from build123d import *

# Parameters (mm, degrees)
BOSS_EXTRU_1_DEPTH     = 200
D_GAGEMENT_M3_52_D     = 4.2
D_GAGEMENT_M3_52_DEPTH = 50
D_GAGEMENT_M3_52_TIP   = 1.2618073


with BuildPart() as part:
    # Esquisse2 → Boss.-Extru.1 (new body)
    with BuildSketch(Plane.XY):
        with BuildLine():
            Line((30, 0), (35, 0))
            Line((35, 0), (35, 10))
            Line((35, 10), (42, 10))
            Line((42, 10), (42, 0))
            Line((42, 0), (50, 0))
            ThreePointArc((50, 0), (35.355339059, 35.355339059), (0, 50))
            Line((0, 50), (0, 42))
            Line((0, 42), (10, 42))
            Line((10, 42), (10, 35))
            Line((10, 35), (0, 35))
            Line((0, 35), (0, 30))
            ThreePointArc((0, 30), (21.213203436, 21.213203436), (30, 0))
        make_face()
    extrude(amount=-BOSS_EXTRU_1_DEPTH)

    # Dégagement M3.52
    with Locations(Plane(origin=(0, 0, -200), x_dir=(-1, 0, 0), z_dir=(0, 0, -1))):
        with Locations((-28.284271247, 28.284271247)):
            Hole(D_GAGEMENT_M3_52_D / 2, depth=D_GAGEMENT_M3_52_DEPTH)
            with Locations((0, 0, -(D_GAGEMENT_M3_52_DEPTH + D_GAGEMENT_M3_52_TIP / 2))):  # 118° drill point
                Cone(0, D_GAGEMENT_M3_52_D / 2, D_GAGEMENT_M3_52_TIP, mode=Mode.SUBTRACT)


solid = part.part
Can you work these out from the model? Positions are in its coordinate system, mm. A direction names the side the tool comes from. Coordinates: 2 decimals unless noted, no trailing zeros. Write each loop counter-clockwise with the first axis right and the second up, starting at its lowest first coordinate (ties: lowest second). Pieces come first, ordered by that corner, then holes.
Q1. If we mould it in two halves opening along Y, with no side actions, what happens to faces 4 (the face through (35.742, 34.964, -98.6)), 5 (the face through (26.736, 29.704, -174.65)), 6 (the face through (38, 10, -99)), 7 (the face through (25, 25, -200))? For each: +Y half, -Y half, draft (parallel to the pull), parting line (faces both ways), or undercut.
Results found:
face 4: +Y half
face 5: undercut
face 6: -Y half
face 7: draft
Q2. Imagine slicing it at C-C, the plane z = -54.5. List the corners of the cut face in (x, y) for me, plus the area to 3 significant figures.
Results found:
outline: (0, 30) arc R30 cw to (30, 0) - (35, 0) - (35, 10) - (42, 10) - (42, 0) - (50, 0) arc R50 ccw to (0, 50) - (0, 42) - (10, 42) - (10, 35) - (0, 35) - close
area: 1,120 mm2
Q3. Imagine slicing it at B-B, the plane z = -153.5. List the corners of the cut face in (x, y) for me, plus the area to 3 significant figures.
Results found:
outline: (0, 30) arc R30 cw to (30, 0) - (35, 0) - (35, 10) - (42, 10) - (42, 0) - (50, 0) arc R50 ccw to (0, 50) - (0, 42) - (10, 42) - (10, 35) - (0, 35) - close; hole circle Ø4.2 at (28.28, 28.28)
area: 1,100 mm2
Q4. Imagine slicing it at A-A, the plane y = 5. List the corners of the cut face in (x, z) for me.
Results found:
outline: (29.58, -200) - (35, -200) - (35, 0) - (29.58, 0) - close; (42, -200) - (49.75, -200) - (49.75, 0) - (42, 0) - close
Q5. For P1, Ø6, axis at x = 25.5, z = -172.5, coming from the +Y side; P2, Ø5, axis at x = 6.5, z = -82, coming from the -Y side; P3, Ø8, axis at y = 6.5, z = -100, coming from the +X side, each with a flat end and sliding along its axis, tell me the tip position at first contact or that it passes through.
Results found:
P1: stops at y = 44.65
P2: stops at y = 28.62
P3: stops at x = 49.94
Q6. Imagine slicing it at D-D, the plane x = 32.5. List the corners of the cut face in (y, z) for me, plus the area to 3 significant figures.
Results found:
outline: (0, -200) - (38, -200) - (38, 0) - (0, 0) - close
area: 7,600 mm2
Q7. Please list where these lines run through material, in increasing order: L1, parallel to X at y = 7, z = -11; L2, parallel to X at y = 2, z = -99.5.
Results found:
L1: x = 29.17 to 35, 42 to 49.51
L2: x = 29.93 to 35, 42 to 49.96
Q8. Which directions (+Z, -Z, +X, -X, +Y, -Y) give clear straight access to the entire face, cutting with the end or side of a thin tool? Please do faces 1 (the face through (28.363, 27.928, -148.957)), 2 (the face through (5, 42, -99)), 3 (the face through (42, 5, -99)).
Results found:
face 1: -Z
face 2: +Z, -Z, -X
face 3: +Z, -Z, -Y
